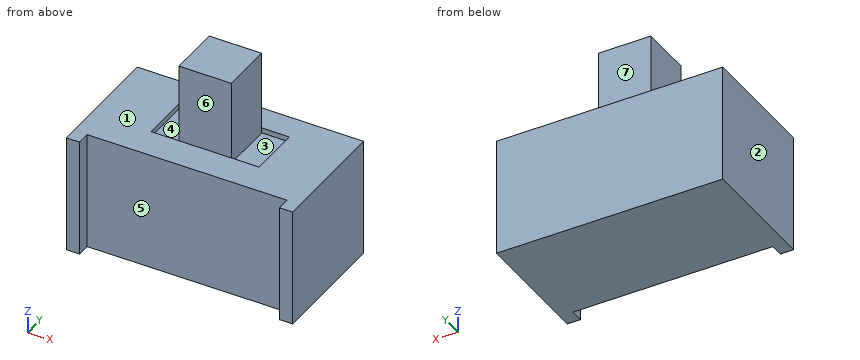
```python
from build123d import *

# Parameters (mm, degrees)
SKETCH_1_W           = 8.6
SKETCH_1_H           = 4.5
EXTRUDE_1_DEPTH      = 4.7
SKETCH_2_W           = 4.1
SKETCH_2_H           = 2
CUT_EXTRUDE_1_DEPTH  = 0.2
CUT_EXTRUDE_2_REACH  = 6.5
SKETCH_4_W           = 7.6
SKETCH_4_H           = 0.5
SKETCH_5_W           = 2
SKETCH_5_H           = 2
EXTRUDE_2_DEPTH      = 3
EXTRUDE_2_DEPTH_BACK = 0.2


with BuildPart() as part:
    # 草图1 → 凸台-拉伸1 (new body)
    with BuildSketch(Plane(origin=(0, 0, 0), x_dir=(1, 0, 0), z_dir=(0, 1, 0))):
        with Locations((4.3, 2.25)):
            Rectangle(SKETCH_1_W, SKETCH_1_H)
    extrude(amount=EXTRUDE_1_DEPTH)

    # 草图2 → 切除-拉伸1 (cut)
    with BuildSketch(Plane.XY):
        with Locations((4.3, 2.7)):
            Rectangle(SKETCH_2_W, SKETCH_2_H)
    extrude(amount=-CUT_EXTRUDE_1_DEPTH, mode=Mode.SUBTRACT)

    # 草图4 → 切除-拉伸2 (cut, up to next)
    with BuildSketch(Plane.XY, mode=Mode.PRIVATE) as cut_extrude_2_sk1:
        with Locations((4.3, 0.25)):
            Rectangle(SKETCH_4_W, SKETCH_4_H)
    cut_extrude_2_tool1 = extrude(cut_extrude_2_sk1.sketch, amount=-CUT_EXTRUDE_2_REACH, mode=Mode.PRIVATE) & part.part
    add(cut_extrude_2_tool1.solids().sort_by_distance((4.3, 0.25, 0))[0], mode=Mode.SUBTRACT)

    # 草图5 → 凸台-拉伸2 (add, two sides)
    with BuildSketch(Plane.XY) as extrude_2_sk:
        with Locations((4.3, 2.7)):
            Rectangle(SKETCH_5_W, SKETCH_5_H)
    extrude(amount=EXTRUDE_2_DEPTH)
    extrude(extrude_2_sk.sketch, amount=-EXTRUDE_2_DEPTH_BACK)


solid = part.part
```
Here's how the part is built. I have some questions about the finished solid (model axes, mm). Face numbers are marked on the shaded views. A direction names the side the tool comes from. Round coordinates to 2 decimals unless told otherwise and drop trailing zeros. Write each loop counter-clockwise with the first axis right and the second up, starting at its lowest first coordinate (ties: lowest second). Pieces come first, ordered by that corner, then holes.
Q1. If we section it at D-D on x = 1.25: Write out the boundary of the cut face in (y, z).
Q2. If we section it at A-A on x = 3: Write out the boundary of the cut face in (y, z), plus the area to 3 significant figures.
Q3. Will these pins go through, and if not, where does the flat tip stop? P1, Ø0.6, axis at x = 4, z = 1.5, coming from the +Y side; P2, Ø0.5, axis at x = 6, y = 3, coming from the +Z side; P3, Ø2.5, axis at x = 3, y = 1, coming from the +Z side; P4, Ø2, axis at x = 4.5, z = 2, coming from the -Y side.
Q4. If we section it at B-B on y = 2.85: Write out the boundary of the cut face in (x, z).
Q5. If we mould it in two halves opening along X, with no side actions, what happens to the marked faces 1, 2 and 3? For each: +X half, -X half, draft (parallel to the pull), parting line (faces both ways), or undercut.
Q6. If we section it at C-C on z = -2: Write out the boundary of the cut face in (x, y), plus the area to 3 significant figures.
Q7. Which directions (+Z, -Z, +X, -X, +Y, -Y) give clear straight access to the entire face, cutting with the end or side of a thin tool? Please do the marked faces 4, 5, 6 and 7.
Q8. Please list where these lines run through material, in increasing order: probe 1 along Z at (x, y) = (6.75, 2.8); probe 2 along X at (y, z) = (3.1, 0.5); probe 3 along Y at (x, z) = (2.25, -2.75).
Answer below:
1. outline: (0.5, -4.5) - (4.7, -4.5) - (4.7, 0) - (0.5, 0) - close
2. outline: (0.5, -4.5) - (4.7, -4.5) - (4.7, 0) - (3.7, 0) - (3.7, -0.2) - (1.7, -0.2) - (1.7, 0) - (0.5, 0) - close
2. area: 18.5 mm2
3. P1: stops at y = 3.7
3. P2: stops at z = -0.2
3. P3: stops at z = 3
3. P4: stops at y = 1.7
4. outline: (0, -4.5) - (8.6, -4.5) - (8.6, 0) - (6.35, 0) - (6.35, -0.2) - (5.3, -0.2) - (5.3, 3) - (3.3, 3) - (3.3, -0.2) - (2.25, -0.2) - (2.25, 0) - (0, 0) - close
5. face 1: draft
5. face 2: -X half
5. face 3: undercut
6. outline: (0, 0) - (0.5, 0) - (0.5, 0.5) - (8.1, 0.5) - (8.1, 0) - (8.6, 0) - (8.6, 4.7) - (0, 4.7) - close
6. area: 36.6 mm2
7. face 4: +Z
7. face 5: +Z, -Z, -Y
7. face 6: +Z, +X, -X, -Y
7. face 7: +Z, +X, -X, +Y
8. probe 1: z = -4.5 to 0
8. probe 2: x = 3.3 to 5.3
8. probe 3: y = 0.5 to 4.7
